Part model, mm, in its own coordinate system. Round coordinates to 2 decimals unless told otherwise and drop trailing zeros. Order: outer loops, then holes, each group sorted by start corner. A loop starts at its lowest first (then second) coordinate and runs counter-clockwise, first axis right, second up. Notation, with made-up numbers: M 49,82.25 L 58,82.25 A20 cw 58,96.25 Z; hole C 31.25,25 d3. An arc over 180 degrees is marked long. Write each question's results on one line, items separated by ' | '. Start each with the question number.
1. Band-saw the part on C-C, the plane z = 0. Give the number of separate pieces and of enclosed holes in the cut face, then the cut area to 3 significant figures.
2. Probe L1, parallel to X at y = 1.95, z = 0; L2, parallel to X at y = 0.7, z = 0; L3, parallel to Z at x = 138.5, y = 1.8. List the from-to ranges inside material, lowest first. Write a range as [from, to].
3. Band-saw the part on A-A, the plane x = 89.5. List the corners of the cut face in (y, z).
4. Drop a flat-ended pin along its axis: pin 1 Ø8 at (x, z) = (120.42, 0) entering from -Y. Give the stop position or say it passes through.
5. Band-saw the part on B-B, the plane x = 135. List the corners of the cut face in (y, z).
6. Band-saw the part on D-D, the plane z = 4.25. List the corners of the cut face in (x, y).
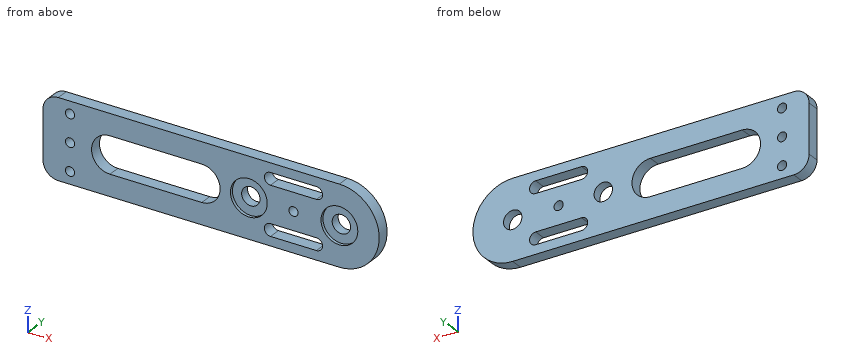
```python
from build123d import *

# Parameters (mm, degrees)
SKETCH_1_R          = 5
SKETCH_1_R_2        = 3
SKETCH_1_R_3        = 1.3
SKETCH_1_R_4        = 1.5
SKETCH_1_W          = 5
SKETCH_1_H          = 10
EXTRUDE_1_DEPTH     = 4
SKETCH_2_R          = 6.01
CUT_EXTRUDE_1_DEPTH = 1
SKETCH_4_W          = 81.277296146
SKETCH_4_H          = 46.186139701
CUT_EXTRUDE_4_DEPTH = 16
FILLET_1_R          = 5


with BuildPart() as part:
    # 草图1 → 凸台-拉伸1 (new body)
    with BuildSketch(Plane(origin=(0, 0, 0), x_dir=(1, 0, 0), z_dir=(0, 1, 0))):
        with BuildLine():
            Line((150, 13), (15.198684154, 13))
            ThreePointArc((15.198684154, 13), (-20, 0), (15.198684154, -13))
            Line((15.198684154, -13), (150, -13))
            ThreePointArc((150, -13), (163, 0), (150, 13))
        make_face()
        with Locations(Location((0, 0, 0), (0, 0, 270))):
            Circle(SKETCH_1_R, mode=Mode.SUBTRACT)
        with Locations(Location((150, 0, 0), (0, 0, 270))):
            Circle(SKETCH_1_R_2, mode=Mode.SUBTRACT)
        with Locations(Location((120.4195, 0, 0), (0, 0, 270))):
            Circle(SKETCH_1_R_2, mode=Mode.SUBTRACT)
        with Locations(Location((0, 9, 0), (0, 0, 270))):
            Circle(SKETCH_1_R_3, mode=Mode.SUBTRACT)
        with Locations(Location((7.794228634, -4.5, 0), (0, 0, 270))):
            Circle(SKETCH_1_R_3, mode=Mode.SUBTRACT)
        with Locations(Location((-7.794228634, -4.5, 0), (0, 0, 270))):
            Circle(SKETCH_1_R_3, mode=Mode.SUBTRACT)
        with Locations(Location((135, 0, 0), (0, 0, 270))):
            Circle(SKETCH_1_R_4, mode=Mode.SUBTRACT)
        with Locations(Location((62, 0, 0), (0, 0, 270))):
            Circle(SKETCH_1_R_4, mode=Mode.SUBTRACT)
        with Locations(Location((62, 9, 0), (0, 0, 270))):
            Circle(SKETCH_1_R_4, mode=Mode.SUBTRACT)
        with Locations(Location((62, -9, 0), (0, 0, 270))):
            Circle(SKETCH_1_R_4, mode=Mode.SUBTRACT)
        with Locations((0, -11.773380776)):
            Rectangle(SKETCH_1_W, SKETCH_1_H, mode=Mode.SUBTRACT)
        with BuildLine():
            Line((105.041482469, -6), (75.041482469, -6))
            ThreePointArc((75.041482469, -6), (69.041482469, 0), (75.041482469, 6))
            Line((75.041482469, 6), (105.041482469, 6))
            ThreePointArc((105.041482469, 6), (111.041482469, 0), (105.041482469, -6))
        make_face(mode=Mode.SUBTRACT)
        with BuildLine():
            Line((142.5, 6), (127.5, 6))
            ThreePointArc((127.5, 6), (125.5, 8), (127.5, 10))
            Line((127.5, 10), (142.5, 10))
            ThreePointArc((142.5, 10), (144.5, 8), (142.5, 6))
        make_face(mode=Mode.SUBTRACT)
        with BuildLine():
            Line((142.5, -6), (127.5, -6))
            ThreePointArc((127.5, -6), (125.5, -8), (127.5, -10))
            Line((127.5, -10), (142.5, -10))
            ThreePointArc((142.5, -10), (144.5, -8), (142.5, -6))
        make_face(mode=Mode.SUBTRACT)
    extrude(amount=EXTRUDE_1_DEPTH)

    # 草图2 → 切除-拉伸1 (cut)
    with BuildSketch(Plane.XZ):
        with Locations(Location((150, 0, 0), (0, 0, 270))):
            Circle(SKETCH_2_R)
        with Locations(Location((120.4195, 0, 0), (0, 0, 270))):
            Circle(SKETCH_2_R)
    extrude(amount=-CUT_EXTRUDE_1_DEPTH, mode=Mode.SUBTRACT)

    # 草图4 → 切除-拉伸4 (cut)
    with BuildSketch(Plane(origin=(0, 4, 0), x_dir=(1, 0, 0), z_dir=(0, 1, 0))):
        with Locations((12.539593114, -0.049090765)):
            Rectangle(SKETCH_4_W, SKETCH_4_H)
    extrude(amount=-CUT_EXTRUDE_4_DEPTH, mode=Mode.SUBTRACT)

    # 圆角1
    fillet_1_edges = [part.edges().sort_by_distance(p)[0] for p in [
        (53.178241187, 2, 13),
        (53.178241187, 2, -13),
    ]]
    fillet(fillet_1_edges, radius=FILLET_1_R)


solid = part.part
```
Solution:
1) separate pieces: 6 | enclosed holes: 0 | area: 187 mm^2
2) L1: [53.18, 60.5], [63.5, 69.04], [111.04, 117.42], [123.42, 133.5], [136.5, 147], [153, 163] | L2: [53.18, 60.5], [63.5, 69.04], [111.04, 114.41], [126.43, 133.5], [136.5, 143.99], [156.01, 163] | L3: [-13, -10], [-6, 6], [10, 13]
3) outline: M 0,-13 L 4,-13 L 4,-6 L 0,-6 Z; M 0,6 L 4,6 L 4,13 L 0,13 Z
4) pin 1: y = 1
5) outline: M 0,-13 L 4,-13 L 4,-10 L 0,-10 Z; M 0,-6 L 4,-6 L 4,-1.5 L 0,-1.5 Z; M 0,1.5 L 4,1.5 L 4,6 L 0,6 Z; M 0,10 L 4,10 L 4,13 L 0,13 Z
6) outline: M 53.18,0 L 70.81,0 L 70.81,4 L 53.18,4 Z; M 109.28,0 L 116.17,0 L 116.17,1 L 124.67,1 L 124.67,0 L 145.75,0 L 145.75,1 L 154.25,1 L 154.25,0 L 162.29,0 L 162.29,4 L 109.28,4 Z
